Check sheet for the modelled part. Datum: model origin and axes. Units: mm. A direction names the side the tool comes from. Round coordinates to 2 decimals unless told otherwise and drop trailing zeros. Write each loop counter-clockwise with the first axis right and the second up, starting at its lowest first coordinate (ties: lowest second). Pieces come first, ordered by that corner, then holes. Notation, with made-up numbers: (80, -5) - (86, -5) arc R20 ccw to (86, 1) - close; hole circle Ø11 at (-39, 74). An arc over 180 degrees is marked (long way). Use one line per item in the form item = value. Start each with the question number.
1) Set-up check for faces 1 (the face through (-0.54, -2.44, 3.96)), 2 (the face through (0, 0, 0)): record each of +Z, -Z, +X, -X, +Y, -Y from which the full face is reachable in a straight line by a thin tool's end or side.
2) Section check C-C (z = 4.75). Record the boundary of the cut face in (x, y), then the cut area to 3 significant figures.
3) Section check D-D (y = -8.5). Record the boundary of the cut face in (x, z).
4) Gauge pin test, flat ends, axial feed: P1, Ø1, axis at x = -16.5, z = 2.5, coming from the +Y side; P2, Ø3, axis at y = 16, z = 2.5, coming from the +X side. Record the tip position at first contact, or that the pin passes through.
5) Section check A-A (x = 0). Record the boundary of the cut face in (y, z).
6) Scan lines: probe 1 along Z at (x, y) = (-5.5, -10.5); probe 2 along Y at (x, z) = (1, 3); probe 3 along Y at (x, z) = (-21, 1.25). Record each from-to range of solid material in increasing order.
7) Section check B-B (y = 0). Record the boundary of the cut face in (x, z), then the cut area to 3 significant figures.
from build123d import *

# Parameters (mm, degrees)
PAD_DEPTH    = 1.5
SKETCH001_R  = 2.5
PAD001_DEPTH = 5


with BuildPart() as part:
    # Sketch → Pad (new body)
    with BuildSketch(Plane.XY):
        with BuildLine():
            Line((17.929835, 14.08407), (17.536637, 13.775209))
            ThreePointArc((17.536637, 13.775209), (8.400618, 20.657193), (-2.94546, 22.104621))
            Line((-3.011501, 22.60024), (-2.94546, 22.104621))
            ThreePointArc((-3.011501, 22.60024), (-21.140537, 8.539186), (-17.863266, -14.168406))
            Line((-17.863266, -14.168406), (-17.471528, -13.857695))
            ThreePointArc((-17.471528, -13.857695), (-8.319433, -20.690023), (3.014889, -22.095258))
            Line((3.014889, -22.095258), (3.082487, -22.590668))
            ThreePointArc((3.082487, -22.590668), (21.133824, -8.555787), (17.929835, 14.08407))
        make_face()
    extrude(amount=PAD_DEPTH)

    # Sketch001 (on Face10 of Pad) → Pad001 (join)
    with BuildSketch(Plane.XY.offset(1.5)):
        Circle(SKETCH001_R)
    extrude(amount=PAD001_DEPTH)


solid = part.part
Results are:
q1.face_1 = +Z
q1.face_2 = -Z, +X, -X, +Y, -Y
q2.outline = circle Ø5 at (0, 0)
q2.area = 19.6 mm²
q3.outline = (-21.16, 0) - (21.16, 0) - (21.16, 1.5) - (-21.16, 1.5) - close
q4.P1 = through
q4.P2 = 16.61
q5.outline = (-22.3, 0) - (22.3, 0) - (22.3, 1.5) - (2.5, 1.5) - (2.5, 6.5) - (-2.5, 6.5) - (-2.5, 1.5) - (-22.3, 1.5) - close
q6.probe_1 = 0 to 1.5
q6.probe_2 = -2.29 to 2.29
q6.probe_3 = -8.88 to 8.88
q7.outline = (-22.8, 0) - (22.8, 0) - (22.8, 1.5) - (2.5, 1.5) - (2.5, 6.5) - (-2.5, 6.5) - (-2.5, 1.5) - (-22.8, 1.5) - close
q7.area = 93.4 mm²
